Part model, mm, in its own coordinate system. Face numbers are marked on the shaded views. A direction names the side the tool comes from. Round coordinates to 2 decimals unless told otherwise and drop trailing zeros. Order: outer loops, then holes, each group sorted by start corner. A loop starts at its lowest first (then second) coordinate and runs counter-clockwise, first axis right, second up. Notation, with made-up numbers: (46.5, 9) - (69.5, 9) arc R15 ccw to (69.5, 38) - close; hole circle Ø2 at (16, 77). An arc over 180 degrees is marked (long way). Return JSON: item names as keys, results as strings. Group by question number.
Item 1: Saw through at C-C on x = 15.5. List the corners of the cut face in (y, z), and give its area (3 significant figures).
Item 2: Saw through at A-A on x = 0. List the corners of the cut face in (y, z), and give its area (3 significant figures).
Item 3: Saw through at B-B on z = 42. List the corners of the cut face in (x, y), and give its area (3 significant figures).
Item 4: Tool access for the marked faces 1 and 2: list every direction of +Z, -Z, +X, -X, +Y, -Y with a clear straight run to the whole face (end or side of a thin tool).
Item 5: Saw through at D-D on y = -9. List the corners of the cut face in (x, z).
Item 6: Drop flat-ended pins along their axis: pin 1 (1.6 mm diameter, centred on y = 16.5, z = 1, fed in from +X); pin 2 (2 mm diameter, centred on y = -16, z = 1, fed in from +X); pin 3 (3 mm diameter, centred on y = 4.5, z = 9.5, fed in from -X). Give the stop position or say it passes through.
Item 7: Probe probe 1 along Y at (x, z) = (24, 42); probe 2 along Y at (x, z) = (0, 1); probe 3 along X at (y, z) = (-11, 5.5). List the from-to ranges inside material, lowest first.
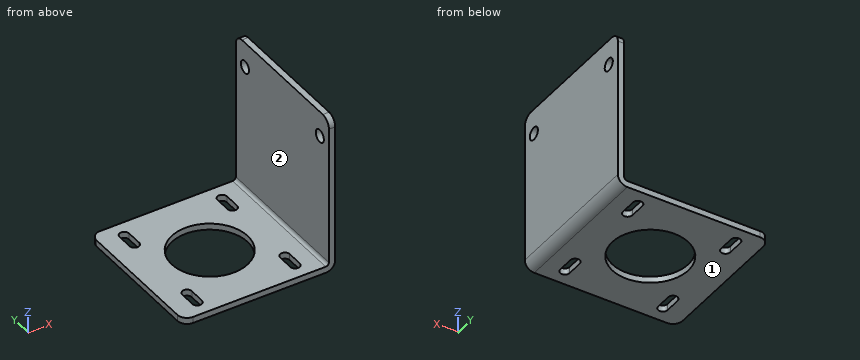
Autodesk Inventor part; units mm, degrees
ref_plane "YZ Plane" through (0, 0, 0) normal (1, 0, 0) x (0, 1, 0)
ref_plane "XZ Plane" through (0, 0, 0) normal (0, 1, 0) x (-1, 0, 0)
ref_plane "XY Plane" through (0, 0, 0) normal (0, 0, 1) x (1, 0, 0)
sketch "Эскиз1" plane through (0, 0, 0) normal (0, 0, 1) x (1, 0, 0)
  circle A0 centre (0, 0) radius 12
  line L0 (0, 0) -> (0, 33) construction
  line L1 (0, 0) -> (-30.4422, 0) construction
  line L2 (-23, 23) -> (25, 23)
  line L3 (25, 23) -> (25, -23)
  line L4 (25, -23) -> (-23, -23)
  line L5 (-23, -23) -> (-23, 23)
  line L6 (15.5, 15.5) -> (-15.5, 15.5) construction
  line L7 (-15.5, 15.5) -> (-15.5, -15.5) construction
  line L8 (15.5, -15.5) -> (15.5, 15.5) construction
  line L9 (-15.5, 15.5) -> (15.5, -15.5) construction
  circle A1 centre (-15.5, 15.5) radius 1.5
  circle A2 centre (15.5, 15.5) radius 1.5
  circle A3 centre (-15.5, -15.5) radius 1.5
  circle A4 centre (15.5, -15.5) radius 1.5
  line L10 (51, 23) -> (51, -23) construction
  line L11 (-25.1704, 23) -> (21, 23) construction
  line L12 (21, -23) -> (-25.1704, -23) construction
  line L13 (-15.5, -13) -> (-15.5, -18) construction
  line L14 (-17, -13) -> (-17, -18)
  line L15 (-14, -18) -> (-14, -13)
  arc A5 (-14, -13) -> (-17, -13) centre (-15.5, -13) ccw
  arc A6 (-17, -18) -> (-14, -18) centre (-15.5, -18) ccw
  line L16 (-15.5, 18) -> (-15.5, 13) construction
  line L17 (-17, 18) -> (-17, 13)
  line L18 (-14, 13) -> (-14, 18)
  arc A7 (-14, 18) -> (-17, 18) centre (-15.5, 18) ccw
  arc A8 (-17, 13) -> (-14, 13) centre (-15.5, 13) ccw
  line L19 (15.5, 18) -> (15.5, 13) construction
  line L20 (14, 18) -> (14, 13)
  line L21 (17, 13) -> (17, 18)
  arc A9 (17, 18) -> (14, 18) centre (15.5, 18) ccw
  arc A10 (14, 13) -> (17, 13) centre (15.5, 13) ccw
  line L22 (15.5, -13) -> (15.5, -18) construction
  line L23 (14, -13) -> (14, -18)
  line L24 (17, -18) -> (17, -13)
  arc A11 (17, -13) -> (14, -13) centre (15.5, -13) ccw
  arc A12 (14, -18) -> (17, -18) centre (15.5, -18) ccw
  dimension "d0" = 24
  dimension "d1" = 31
  dimension "d2" = 31
  dimension "d3" = 3
  dimension "d4" = 3
  dimension "d5" = 3
  dimension "d6" = 3
  dimension "d7" = 46
  dimension "d51" = 48
  dimension "d52" = 23
  dimension "d53" = 8
  dimension "d54" = 8
  dimension "d55" = 8
  dimension "d56" = 8
extrude "Выдавливание4" add sketch "Эскиз1" along normal blind 2
sketch "Эскиз3" plane through (0, 0, 2) normal (0, 0, 1) x (1, 0, 0)
  line L0 (25, -23) -> (23, -23)
  line L1 (23, -23) -> (23, 23)
  line L2 (23, 23) -> (25, 23)
  line L3 (25, 23) -> (25, -23)
  line L4 (-23, 23) -> (-23, -23)
  line L5 (25, -23) -> (-23, -23)
  line L6 (-23, 23) -> (25, 23)
  line L7 (25, -23) -> (25, 23)
  point P0 (0, 0)
  dimension "d32" = 2
extrude "Выдавливание5" add sketch "Эскиз3" along normal blind 48 contours L0 L1 L2 L3
sketch "Эскиз4" plane through (23, -23, 2) normal (-1, 0, 0) x (0, 0, 1)
  line L0 (40, 4.5) -> (40, 41.5) construction
  circle A0 centre (40, 41.5) radius 2
  circle A1 centre (40, 4.5) radius 2
  line L1 (0, 41) -> (0, 1)
  line L2 (48, 46) -> (48, 0)
  line L3 (48, 23) -> (59.018, 23)
  point P0 (20, 21)
  dimension "d42" = 4
  dimension "d43" = 4
  dimension "d50" = 37
  dimension "d60" = 8
extrude "Выдавливание6" cut sketch "Эскиз4" against normal blind 10
fillet "Сопряжение2" radius 1 1 edges at (23, 0, 2)
fillet "Сопряжение3" radius 3 1 edges at (25, 0, 0)
fillet "Сопряжение4" radius 3 4 edges at (-23, -23, 1) (-23, 23, 1) (24, 23, 50) (24, -23, 50)
properties part number "Plastina  motor"
Filled in:
{
 "1": {"outline": "(-23, 0) - (-19.5, 0) - (-19.5, 2) - (-23, 2) - close; (-11.5, 0) - (11.5, 0) - (11.5, 2) - (-11.5, 2) - close; (19.5, 0) - (23, 0) - (23, 2) - (19.5, 2) - close", "area": "60.0 mm^2"},
 "2": {"outline": "(-23, 0) - (-12, 0) - (-12, 2) - (-23, 2) - close; (12, 0) - (23, 0) - (23, 2) - (12, 2) - close", "area": "44.0 mm^2"},
 "3": {"outline": "(23, -23) - (25, -23) - (25, -20.5) - (23, -20.5) - close; (23, -16.5) - (25, -16.5) - (25, 16.5) - (23, 16.5) - close; (23, 20.5) - (25, 20.5) - (25, 23) - (23, 23) - close", "area": "76.0 mm^2"},
 "4": {"face 1": "-Z, +X, -X, +Y, -Y", "face 2": "+Z, -X, +Y, -Y"},
 "5": {"outline": "(-23, 0) - (-7.94, 0) - (-7.94, 2) - (-23, 2) - close; (7.94, 0) - (22, 0) arc R3 ccw to (25, 3) - (25, 50) - (23, 50) - (23, 3) arc R1 cw to (22, 2) - (7.94, 2) - close"},
 "6": {"pin 1": "stops at x = 24.75", "pin 2": "stops at x = 24.83", "pin 3": "stops at x = 23"},
 "7": {"probe 1": "y = -23 to -20.5, -16.5 to 16.5, 20.5 to 23", "probe 2": "y = -23 to -12, 12 to 23", "probe 3": "x = 23 to 25"}
}
